Could you check a few things on this drawing? It's one solid part, dimensions in mm from its lowest x, y, z. A direction names the side the tool comes from. Give positions to 0.01 mm unless a question says otherwise; leave off trailing zeros. Order: outer loops, then holes, each group sorted by start corner. A loop starts at its lowest first (then second) coordinate and runs counter-clockwise, first axis right, second up.
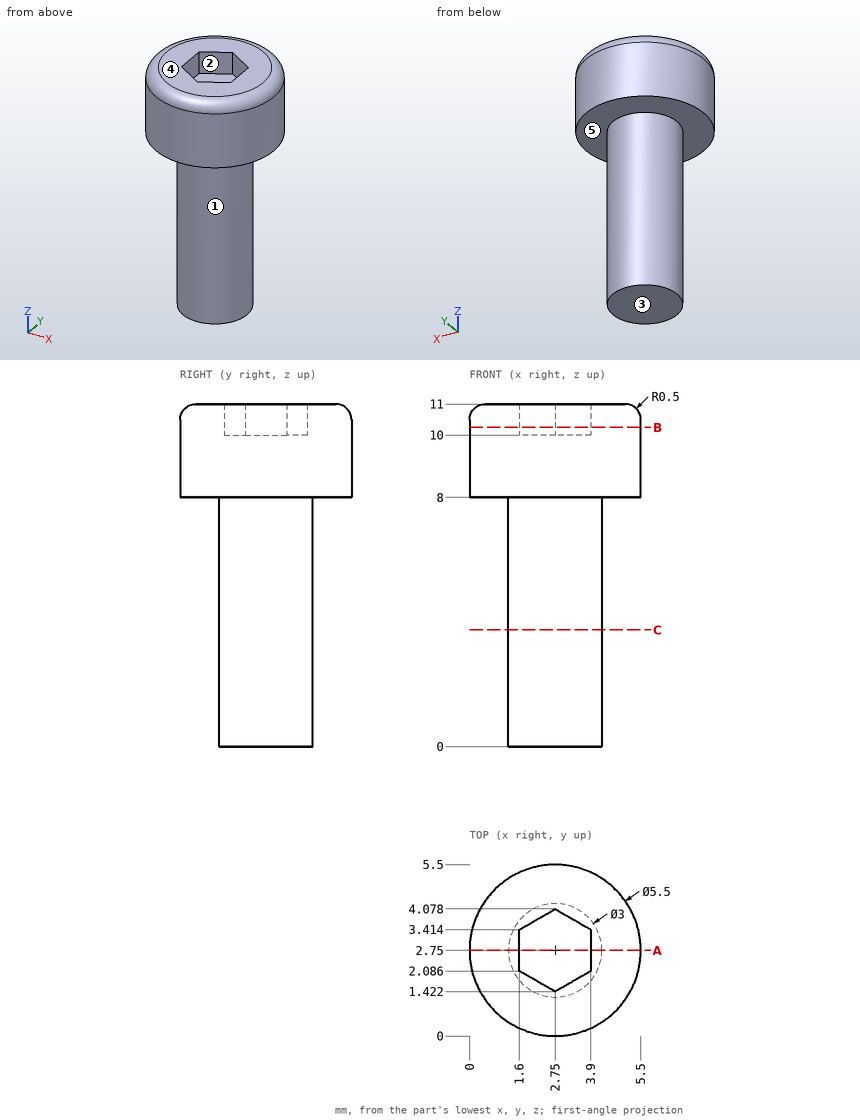
Item 1: Imagine slicing it at A-A on y = 2.75. List the corners of the cut face in (x, z) for me, then the cut area to 3 significant figures.
Findings:
outline: (0, 8) - (1.25, 8) - (1.25, 0) - (4.25, 0) - (4.25, 8) - (5.5, 8) - (5.5, 10.5) arc R0.5 ccw to (5, 11) - (3.9, 11) - (3.9, 10) - (1.6, 10) - (1.6, 11) - (0.5, 11) arc R0.5 ccw to (0, 10.5) - close
area: 38.1 mm2
Item 2: We'd pull the mould along Y, two halves only. Please class the marked faces 1, 2 and 3: +Y half, -Y half, draft (parallel to the pull), parting line (faces both ways), or undercut.
Findings:
face 1: parting line
face 2: undercut
face 3: draft
Item 3: Please list where these lines run through material, in increasing order: line 1 along Z through (x, y) = (2.5, 4.5); line 2 along X through (y, z) = (3.3, 10.5); line 3 along Z through (x, y) = (3.4, 2.6).
Findings:
line 1: z = 8 to 11
line 2: x = 0.06 to 1.6, 3.9 to 5.44
line 3: z = 0 to 10
Item 4: Imagine slicing it at B-B on z = 10.25. List the corners of the cut face in (x, y) for me.
Findings:
outline: circle Ø5.5 at (2.75, 2.75); hole (1.6, 2.09) - (2.75, 1.42) - (3.9, 2.09) - (3.9, 3.41) - (2.75, 4.08) - (1.6, 3.41) - close
Item 5: Imagine slicing it at C-C on z = 3.75. List the corners of the cut face in (x, y) for me, then the cut area to 3 significant figures.
Findings:
outline: circle Ø3 at (2.75, 2.75)
area: 7.07 mm2
Item 6: For pin 1 (0.5 mm diameter, centred on y = 3, z = 10.5, fed in from +X); pin 2 (1 mm diameter, centred on y = 5, z = 9, fed in from +X), each with a flat end and sliding along its axis, tell me the tip position at first contact or that it passes through.
Findings:
pin 1: stops at x = 5.5
pin 2: stops at x = 4.87
Item 7: For the marked faces 4 and 5, which set-ups out of +Z, -Z, +X, -X, +Y, -Y let a thin tool reach every point of the face, with its end or its side?
Findings:
face 4: +Z, +X, -X, +Y, -Y
face 5: -Z
